Could you check a few things on this model? Use its own coordinates, in mm. Face numbers are marked on the shaded views. A direction names the side the tool comes from. Give positions to 0.01 mm unless a question says otherwise; leave off trailing zeros. Order: outer loops, then holes, each group sorted by start corner. A loop starts at its lowest first (then second) coordinate and runs counter-clockwise, first axis right, second up.
(1) If we mould it in two halves opening along X, with no side actions, what happens to the marked faces 3, 4 and 5? For each: released by +X, released by -X, zero draft, split by the parting line, or undercut.
(2) Imagine slicing it at B-B, the plane z = -15. Write out the boundary of the cut face in (x, y).
(3) On a 3-axis mill with a long thin cutter (end or side, diameter ignored), from which of +Z, -Z, +X, -X, +Y, -Y can I reach the whole of each face in a straight line? I mean the marked faces 1 and 2. Say none if no direction works.
(4) If I drill on probe 1 along X at (y, z) = (4.6, -13.75); probe 2 along X at (y, z) = (1.1, -11.5); probe 3 along Z at (x, y) = (29.5, 2.75), over which ranges is the centre line in solid material (lowest first)?
(5) Imagine slicing it at A-A, the plane x = 26.5. Write out the boundary of the cut face in (y, z), then the cut area to 3 significant figures.
(6) Imagine slicing it at C-C, the plane y = 2. Write out the boundary of the cut face in (x, z), then the cut area to 3 significant figures.
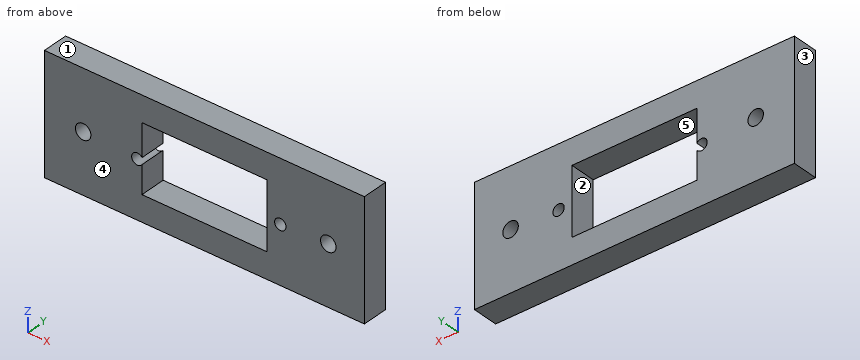
from build123d import *

# Parameters (mm, degrees)
SKETCH4_W           = 62
SKETCH4_H           = 23
SKETCH4_W_2         = 24.2
SKETCH4_H_2         = 13
BOSS_EXTRUDE2_DEPTH = 5
SKETCH7_R           = 1.1
SKETCH7_R_2         = 1.5
CUT_EXTRUDE3_DEPTH  = 10


with BuildPart() as part:
    # Sketch4 → Boss-Extrude2 (new body)
    with BuildSketch(Plane(origin=(0, 0, 0), x_dir=(1, 0, 0), z_dir=(0, 1, 0))):
        with Locations((31, 11.5)):
            Rectangle(SKETCH4_W, SKETCH4_H)
        with Locations((31, 11.5)):
            Rectangle(SKETCH4_W_2, SKETCH4_H_2, mode=Mode.SUBTRACT)
    extrude(amount=BOSS_EXTRUDE2_DEPTH)

    # Sketch7 → Cut-Extrude3 (cut)
    with BuildSketch(Plane(origin=(0, 5, 0), x_dir=(1, 0, 0), z_dir=(0, 1, 0))):
        with Locations(Location((45.7, 11.95, 0), (0, 0, 270))):
            Circle(SKETCH7_R)
        with Locations((18, 11.95)):
            Circle(SKETCH7_R)
        with Locations(Location((7.5, 11.5, 0), (0, 0, 270))):
            Circle(SKETCH7_R_2)
        with Locations(Location((55, 11.5, 0), (0, 0, 270))):
            Circle(SKETCH7_R_2)
    extrude(amount=-CUT_EXTRUDE3_DEPTH, mode=Mode.SUBTRACT)


solid = part.part
Answer block:
1. face 3: released by -X
1. face 4: zero draft
1. face 5: undercut
2. outline: (0, 0) - (18.9, 0) - (18.9, 5) - (0, 5) - close; (43.1, 0) - (62, 0) - (62, 5) - (43.1, 5) - close
3. face 1: +Z, +X, -X, +Y, -Y
3. face 2: +Y, -Y
4. probe 1: x = 0 to 18.9, 43.1 to 62
4. probe 2: x = 0 to 6, 9 to 17, 43.1 to 44.7, 46.7 to 53.5, 56.5 to 62
4. probe 3: z = -23 to -18, -5 to 0
5. outline: (0, -23) - (5, -23) - (5, -18) - (0, -18) - close; (0, -5) - (5, -5) - (5, 0) - (0, 0) - close
5. area: 50.0 mm2
6. outline: (0, -23) - (62, -23) - (62, 0) - (0, 0) - close; hole circle Ø3 at (7.5, -11.5); hole (18.9, -18) - (43.1, -18) - (43.1, -5) - (18.9, -5) - (18.9, -11.32) arc R1.1 ccw (long way) to (18.9, -12.58) - close; hole circle Ø2.2 at (45.7, -11.95); hole circle Ø3 at (55, -11.5)
6. area: 1,090 mm2
